Design review of the part built by this model. Coordinates are the model's own, in mm. Coordinates: 2 decimals unless noted, no trailing zeros. Loops run counter-clockwise (first coordinate to the right, second up) from the corner with the lowest first, then second, coordinate; pieces in that order, holes last. Notation, with made-up numbers: (47, -11.5) -> (57, -11.5) arc R24 cw to (57, 15.5) -> close; hole circle Ø8 at (-7, 84). An arc over 180 degrees is marked (long way). Use a Markdown table: item, result. Add a question column.
Q1. Take a section at B-B on x = -44. Write out the cut boundary in (y, z), plus the area to 3 significant figures.
Q2. Take a section at C-C on z = -20.5. Write out the cut boundary in (x, y).
Q3. Clearance check with flat-ended pins moving along their axes: pin 1 Ø1.6 at (x, y) = (-24.5, 2) entering from +Z; pin 2 Ø1.5 at (x, y) = (-92, 2) entering from -Z; pin 3 Ø1.5 at (y, z) = (1, 29.5) entering from +X. State where each tip first meets the part, or that it passes through.
Q4. Take a section at A-A on y = 0.7. Count the separate pieces of the cut face and the enclosed holes in it, plus the area to 3 significant figures.
Q5. For probe 1 along X at (y, z) = (0.8, 27.5); probe 2 along Z at (x, y) = (-59.5, 0.2); probe 3 along Z at (x, y) = (-45, 2.9), list the stretches that pass through material, from the lowest coordinate up.
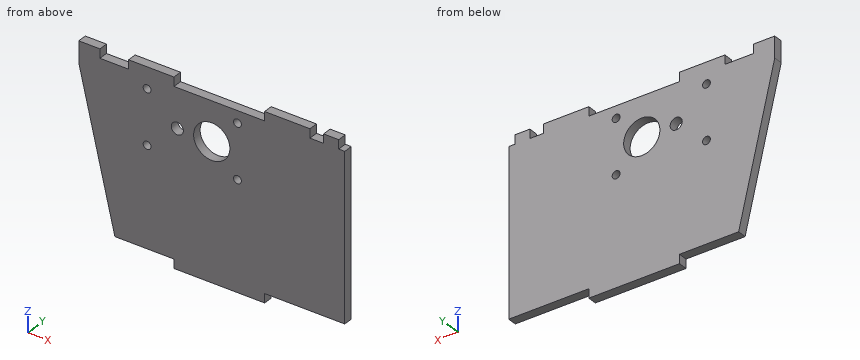
from build123d import *

# Parameters (mm, degrees)
SKETCH1_R           = 2
SKETCH1_R_2         = 6
SKETCH1_R_3         = 1.3
BOSS_EXTRUDE1_DEPTH = 3


with BuildPart() as part:
    # Sketch1 → Boss-Extrude1 (new body)
    with BuildSketch(Plane(origin=(0, 0, 0), x_dir=(1, 0, 0), z_dir=(0, 1, 0))):
        Polygon((-95.483372271, 27.767651072), (-80.483372271, 27.767651072), (-80.483372271, 30.767651072), (-50.483372271, 30.767651072), (-50.483372271, 27.767651072), (-35.483372271, 27.767651072), (-25.983372271, 27.767651072), (-23.983372271, 27.767651072), (-23.983372271, -27.232348928), (-25.983372271, -27.232348928), (-25.983372271, -30.232348928), (-30.983372271, -30.232348928), (-30.983372271, -27.232348928), (-35.483372271, -27.232348928), (-35.483372271, -30.232348928), (-50.483372271, -30.232348928), (-50.483372271, -27.232348928), (-80.483372271, -27.232348928), (-80.483372271, -30.232348928), (-95.483372271, -30.232348928), (-95.483372271, -27.232348928), (-104.983372271, -27.232348928), (-104.983372271, -30.232348928), (-111.983372271, -30.232348928), (-111.983372271, -27.232348928), (-111.983372271, -23.232348928), (-100.033372271, 27.767651072), align=None)
        with Locations(Location((-79.383372271, -14.232348928, 0), (0, 0, 270))):
            Circle(SKETCH1_R, mode=Mode.SUBTRACT)
        with Locations(Location((-67.983372271, -14.232348928, 0), (0, 0, 270))):
            Circle(SKETCH1_R_2, mode=Mode.SUBTRACT)
        with Locations(Location((-59.483372271, -23.232348928, 0), (0, 0, 270))):
            Circle(SKETCH1_R_3, mode=Mode.SUBTRACT)
        with Locations(Location((-59.483372271, -5.232348928, 0), (0, 0, 270))):
            Circle(SKETCH1_R_3, mode=Mode.SUBTRACT)
        with Locations(Location((-89.383372271, -5.232348928, 0), (0, 0, 270))):
            Circle(SKETCH1_R_3, mode=Mode.SUBTRACT)
        with Locations(Location((-89.383372271, -23.232348928, 0), (0, 0, 270))):
            Circle(SKETCH1_R_3, mode=Mode.SUBTRACT)
    extrude(amount=BOSS_EXTRUDE1_DEPTH)


solid = part.part
Answer list:
| question | item | result |
|---|---|---|
| 1 | outline | (0, -27.77) -> (3, -27.77) -> (3, 30.23) -> (0, 30.23) -> close |
| 1 | area | 174 mm² |
| 2 | outline | (-101.74, 0) -> (-23.98, 0) -> (-23.98, 3) -> (-101.74, 3) -> close |
| 3 | pin 1 | z = 27.23 |
| 3 | pin 2 | z = -27.77 |
| 3 | pin 3 | x = -25.98 |
| 4 | separate pieces | 1 |
| 4 | enclosed holes | 6 |
| 4 | area | 4,600 mm² |
| 5 | probe 1 | -111.98 to -104.98, -95.48 to -80.48, -50.48 to -35.48, -30.98 to -25.98 |
| 5 | probe 2 | -30.77 to 3.93, 6.53 to 21.93, 24.53 to 27.23 |
| 5 | probe 3 | -27.77 to 30.23 |
